Could you check a few things on this model? Use its own coordinates, in mm. A direction names the side the tool comes from. Give positions to 0.01 mm unless a question says otherwise; leave off trailing zeros. Order: outer loops, then holes, each group sorted by start corner. A loop starts at its lowest first (then second) coordinate and runs counter-clockwise, first axis right, second up. Notation, with made-up numbers: (58, -24.5) -> (65, -24.5) arc R22 ccw to (65, 6.5) -> close; hole circle Ø11 at (-34, -7). An arc over 180 degrees is marked (long way). Write each question's results on one line, items separated by ' | '.
```python
from build123d import *

# Parameters (mm, degrees)
SKETCH_R           = 31
PAD_DEPTH          = 4
SKETCH002_R        = 11.3
POCKET001_DEPTH    = 4.001
SKETCH004_R        = 2.1
POCKET002_DEPTH    = 179.545866
SKETCH005_R        = 1.6
POCKET003_DEPTH    = 4.001
POLARPATTERN_COUNT = 2
CHAMFER_SIZE       = 1.5
CHAMFER001_SIZE    = 1.5


with BuildPart() as part:
    # Sketch → Pad (new body)
    with BuildSketch(Plane.XY):
        Circle(SKETCH_R)
    extrude(amount=PAD_DEPTH)

    # Sketch002 (on Face3 of Pad) → Pocket001 (cut, through all)
    with BuildSketch(Plane.XY.offset(4)):
        Circle(SKETCH002_R)
    extrude(amount=-POCKET001_DEPTH, mode=Mode.SUBTRACT)

    # Sketch004 (on Face3 of Pocket001) → Pocket002 (cut, through all)
    with BuildSketch(Plane.XY.offset(4)):
        with Locations((-25, 0)):
            Circle(SKETCH004_R)
    pocket002 = extrude(amount=-POCKET002_DEPTH, mode=Mode.SUBTRACT)

    # Sketch005 → Pocket003 (cut, through all)
    with BuildSketch(Plane(origin=(0, 0, 0), x_dir=(1, 0, 0), z_dir=(0, 0, -1))):
        with Locations((0, 11.25)):
            Circle(SKETCH005_R)
    extrude(amount=-POCKET003_DEPTH, mode=Mode.SUBTRACT)

    # PolarPattern: Pocket002 ×2 about axis
    polarpattern_axis = Axis((0, 0, 4), (0, 0, 1))
    for i in range(1, POLARPATTERN_COUNT):
        add(pocket002.rotate(polarpattern_axis, i * 360 / POLARPATTERN_COUNT), mode=Mode.SUBTRACT)

    # Chamfer
    chamfer_edges = [part.edges().sort_by_distance(p)[0] for p in [
        (-31, 0, 4),
    ]]
    chamfer(chamfer_edges, length=CHAMFER_SIZE)

    # Chamfer001
    chamfer001_edges = [part.edges().sort_by_distance(p)[0] for p in [
        (27.1, 0, 4),
        (-27.1, 0, 4),
    ]]
    chamfer(chamfer001_edges, length=CHAMFER001_SIZE)


solid = part.part
```
Q1. Suppose I cut it at A-A on x = 0. Please give me the cut outline in (y, z).
Here are the results:
outline: (-31, 0) -> (-12.85, 0) -> (-12.85, 4) -> (-29.5, 4) -> (-31, 2.5) -> close; (11.3, 0) -> (31, 0) -> (31, 2.5) -> (29.5, 4) -> (11.3, 4) -> close
Q2. Suppose I cut it at C-C on z = 0.75. Please give me the cut outline in (x, y), and give its area (3 significant figures).
Here are the results:
outline: circle Ø62 at (0, 0); hole circle Ø4.2 at (-25, 0); hole (-1.6, -11.19) arc R1.6 ccw (long way) to (1.6, -11.19) arc R11.3 ccw (long way) to start; hole circle Ø4.2 at (25, 0) | area: 2,590 mm²
Q3. Suppose I cut it at B-B on y = 0. Please give me the cut outline in (x, z).
Here are the results:
outline: (-31, 0) -> (-27.1, 0) -> (-27.1, 2.5) -> (-28.6, 4) -> (-29.5, 4) -> (-31, 2.5) -> close; (-22.9, 0) -> (-11.3, 0) -> (-11.3, 4) -> (-21.4, 4) -> (-22.9, 2.5) -> close; (11.3, 0) -> (22.9, 0) -> (22.9, 2.5) -> (21.4, 4) -> (11.3, 4) -> close; (27.1, 0) -> (31, 0) -> (31, 2.5) -> (29.5, 4) -> (28.6, 4) -> (27.1, 2.5) -> close
Q4. I'm going to push flat-ended pins straight in: pin 1 Ø5 at (x, y) = (25, 0) entering from -Z; pin 2 Ø5 at (x, y) = (-25, 0) entering from +Z; pin 3 Ø2 at (x, z) = (23.5, 1) entering from -Y; pin 4 Ø1 at (y, z) = (-2.5, 1) entering from +X. Where does each tip first touch, or does it pass through?
Here are the results:
pin 1: stops at z = 0 | pin 2: stops at z = 2.9 | pin 3: stops at y = -21.32 | pin 4: stops at x = 30.94
Q5. Thinking about a two-plate mould opening in X: for faces 3 (the cylindrical face through (-4.036, 30.736, 1.232)), 4 (the cylindrical face through (0.47, 11.29, 2.03)), 5 (the cylindrical face through (22.997, -0.631, 1.268)), 6 (the flat face through (13, 0, 4)), which applies, +X half, -X half, draft (parallel to the pull), parting line (faces both ways), or undercut?
Here are the results:
face 3: parting line | face 4: undercut | face 5: undercut | face 6: draft
Q6. I need wall thicknesses on line 1 along Y through (x, z) = (0, 2.45); line 2 along Y through (x, z) = (-21, 3.5); line 3 along X through (y, z) = (2, 2.65). Which ranges of each line are inside material? Lowest first, please.
Here are the results:
line 1: y = -31 to -12.85, 11.3 to 31 | line 2: y = -21.42 to 21.42 | line 3: x = -30.79 to -26.03, -23.97 to -11.12, 11.12 to 23.97, 26.03 to 30.79
Q7. For faces 1 (the flat face through (0, -13, 0)), 2 (the cylindrical face through (0.04, -12.85, 1.97)), which set-ups out of +Z, -Z, +X, -X, +Y, -Y let a thin tool reach every point of the face, with its end or its side?
Here are the results:
face 1: -Z, +X, -X, +Y, -Y | face 2: +Z, -Z
